```python
from build123d import *

# Parameters (mm, degrees)
F0_R     = 22.225
F0_R_2   = 14.2875
F0_R_3   = 9.525
F1_DEPTH = 12.7


# Not quite as in the source:
# - the program builds the solid bodies; features that only make, move or delete a surface that nothing else refers to are left out


with BuildPart() as f1:
    # F0 (on Front) → F1 (new body, symmetric)
    with BuildSketch(Plane.XZ):
        with BuildLine():
            ThreePointArc((0.3447838863, 54.6782803896), (1.274446594, 51.2059603319), (1.5875, 47.625))
            ThreePointArc((1.5875, 47.625), (-19.05, 26.9875), (-39.6875, 47.625))
            ThreePointArc((-39.6875, 47.625), (-53.8375681408, 28.2490113175), (-75.9968, 19.05))
            Line((-75.9968, 19.05), (-63.2968, 19.05))
            ThreePointArc((-63.2968, 19.05), (-44.2468, 0), (-63.2968, -19.05))
            Line((-63.2968, -19.05), (-88.6968, -19.05))
            Line((-88.6968, -19.05), (-6.3772739602, -34.3378468245))
            ThreePointArc((-6.3772739602, -34.3378468245), (-3.2021232024, -34.7779019434), (0, -34.925))
            ThreePointArc((0, -34.925), (14.789161423, -31.6391581652), (26.7955113754, -22.3999150697))
            ThreePointArc((26.7955113754, -22.3999150697), (26.830059594, -22.3587292729), (26.8647470812, -22.3176607024))
            ThreePointArc((26.8647470812, -22.3176607024), (36.4241213525, -16.9130263167), (47.2042520761, -19.005988544))
            ThreePointArc((47.2042520761, -19.005988544), (69.6313679155, -19.3648496329), (80.9498, 0))
            ThreePointArc((80.9498, 0), (76.0683727679, 27.6867119276), (62.0118668229, 52.0341345797))
            ThreePointArc((62.0118668229, 52.0341345797), (42.3521205548, 59.8164947236), (25.0767563288, 47.625))
            ThreePointArc((25.0767563288, 47.625), (10.9100684584, 44.8375705557), (0.3447838863, 54.6782803896))
        make_face()
        Circle(F0_R, mode=Mode.SUBTRACT)
        with BuildLine():
            Line((-63.2968, 19.05), (-75.9968, 19.05))
            Line((-75.9968, 19.05), (-88.6968, 19.05))
            ThreePointArc((-88.6968, 19.05), (-107.7468, 0), (-88.6968, -19.05))
            Line((-88.6968, -19.05), (-63.2968, -19.05))
            ThreePointArc((-63.2968, -19.05), (-44.2468, 0), (-63.2968, 19.05))
        make_face()
        with BuildLine():
            ThreePointArc((-88.6968, -11.0998), (-99.7966, 0), (-88.6968, 11.0998))
            Line((-88.6968, 11.0998), (-63.2968, 11.0998))
            ThreePointArc((-63.2968, 11.0998), (-52.197, 0), (-63.2968, -11.0998))
            Line((-63.2968, -11.0998), (-88.6968, -11.0998))
        make_face(mode=Mode.SUBTRACT)
        Circle(F0_R)
        Circle(F0_R_2, mode=Mode.SUBTRACT)
        with BuildLine():
            ThreePointArc((-39.6875, 47.625), (-19.05, 26.9875), (1.5875, 47.625))
            ThreePointArc((1.5875, 47.625), (1.274446594, 51.2059603319), (0.3447838863, 54.6782803896))
            ThreePointArc((0.3447838863, 54.6782803896), (-22.6309603319, 67.949446594), (-39.6875, 47.625))
        make_face()
        with Locations((-19.05, 47.625)):
            Circle(F0_R_3, mode=Mode.SUBTRACT)
    extrude(amount=F1_DEPTH, both=True)


solid = f1.part
```
Read the model definition and answer for the solid it produces. Units are mm, in the model's axes. A direction names the side the tool comes from. Give positions to 0.01 mm unless a question says otherwise; leave off trailing zeros. Loops run counter-clockwise (first coordinate to the right, second up) from the corner with the lowest first, then second, coordinate; pieces in that order, holes last.
Item 1: The part is cut by section B-B (y = 6). Give the number of separate pieces and of enclosed holes in the cut face, and give its area (3 significant figures).
Item 2: The mould has two halves that part along Z. Classify faces 3 (the cylindrical face through (-99.794, -0.178, -0.244)), 4 (the cylindrical face through (69.343, -0.178, -19.524)), 5 (the flat face through (-82, 0, 19.05)), 6 (the cylindrical face through (-52.2, -0.2, 0.2)): released by +Z, released by -Z, zero draft, split by the parting line, or undercut.
Item 3: Find the intervals of material crossed by line 1 along Z through (x, y) = (-11, 3.75); line 2 along X through (y, z) = (8, 9); line 3 along X through (y, z) = (1.5, -1.5), in increasing order.
Item 4: For faces 1 (the flat face through (-76, 0, -11.1)), 2 (the cylindrical face through (42.66, -0.18, 59.85)), determine the directions among +Z, -Z, +X, -X, +Y, -Y from which every point of the face is accessible in a straight line to the end or side of a thin tool.
Item 5: The part is cut by section A-A (x = -19.05). Write down the section's boundary in (y, z).
Item 6: The part is cut by section C-C (z = 31). Write down the section's boundary in (x, y).
Item 7: Each of these flat-tipped pins is pushed along its axis until it touches: pin 1 Ø4 at (y, z) = (-0.5, 45.5) entering from -X; pin 2 Ø5 at (y, z) = (-7.5, 43.5) entering from -X; pin 3 Ø17 at (x, z) = (0, 0) entering from -Y; pin 4 Ø3 at (y, z) = (2.5, 38.5) entering from +X. Where does it stop, or does it pass through?
Item 8: The part is cut by section D-D (x = -48). Write down the section's boundary in (y, z), and give its area (3 significant figures).
Taken from the geometry:
1. separate pieces: 1
1. enclosed holes: 3
1. area: 10,700 mm2
2. face 3: undercut
2. face 4: released by -Z
2. face 5: released by +Z
2. face 6: undercut
3. line 1: z = -33.48 to -9.12, 9.12 to 42.53, 52.72 to 66.63
3. line 2: x = -105.49 to -95.19, -56.8 to -11.1, 11.1 to 80.45
3. line 3: x = -107.69 to -99.69, -52.3 to -14.21, 14.21 to 80.9
4. face 1: +Y, -Y
4. face 2: +Z, +Y, -Y
5. outline: (-12.7, -31.98) - (12.7, -31.98) - (12.7, 38.1) - (-12.7, 38.1) - close; (-12.7, 57.15) - (12.7, 57.15) - (12.7, 68.26) - (-12.7, 68.26) - close
6. outline: (-50.66, -12.7) - (74.78, -12.7) - (74.78, 12.7) - (-50.66, 12.7) - close
7. pin 1: stops at x = -41.47
7. pin 2: stops at x = -42.81
7. pin 3: passes through
7. pin 4: stops at x = 72
8. outline: (-12.7, -26.61) - (12.7, -26.61) - (12.7, 33.77) - (-12.7, 33.77) - close
8. area: 1,530 mm2
